Work out the finished part from the listing and answer in its coordinate system (mm). A direction names the side the tool comes from. Round coordinates to 2 decimals unless told otherwise and drop trailing zeros. Write each loop counter-clockwise with the first axis right and the second up, starting at its lowest first coordinate (ties: lowest second). Pieces come first, ordered by that corner, then holes. Notation, with made-up numbers: M 76,48.5 L 108,48.5 A19 ccw 108,54.5 Z; hole C -38.75,68.5 d9. An arc over 180 degrees is marked long. Answer in a Markdown table with one row per item.
```python
from build123d import *

# Parameters (mm, degrees)
BOSS_EXTRUDE1_DEPTH = 30
FILLET1_R           = 2
SHELL2_T            = 6
SKETCH3_R           = 9
CUT_EXTRUDE1_DEPTH  = 10
SKETCH4_R           = 9
CUT_EXTRUDE2_DEPTH  = 10
SKETCH5_R           = 9
CUT_EXTRUDE3_DEPTH  = 10
SKETCH7_R           = 4.5
CUT_EXTRUDE4_DEPTH  = 10
SKETCH8_R           = 4.5
CUT_EXTRUDE5_DEPTH  = 10
SKETCH9_R           = 4.5
CUT_EXTRUDE6_DEPTH  = 10
CHAMFER2_SIZE       = 2.5


with BuildPart() as part:
    # Sketch1 → Boss-Extrude1 (new body)
    with BuildSketch(Plane.XY):
        with BuildLine():
            Line((2, 0), (28, 0))
            ThreePointArc((28, 0), (29.414213562, 0.585786438), (30, 2))
            Line((30, 2), (30, 28))
            ThreePointArc((30, 28), (29.414213562, 29.414213562), (28, 30))
            Line((28, 30), (2, 30))
            ThreePointArc((2, 30), (0.585786438, 29.414213562), (0, 28))
            Line((0, 28), (0, 2))
            ThreePointArc((0, 2), (0.585786438, 0.585786438), (2, 0))
        make_face()
    extrude(amount=BOSS_EXTRUDE1_DEPTH)

    # Fillet1
    fillet1_edges = [part.edges().sort_by_distance(p)[0] for p in [
        (29.414213562, 0.585786438, 30),
        (15, 0, 0),
        (0.585786438, 0.585786438, 0),
        (30, 15, 30),
        (29.414213562, 29.414213562, 30),
        (15, 30, 30),
        (0.585786438, 29.414213562, 30),
        (0, 15, 30),
        (0.585786438, 0.585786438, 30),
        (15, 0, 30),
        (0, 15, 0),
        (0.585786438, 29.414213562, 0),
        (15, 30, 0),
        (29.414213562, 29.414213562, 0),
        (30, 15, 0),
        (29.414213562, 0.585786438, 0),
    ]]
    fillet(fillet1_edges, radius=FILLET1_R)

    # Shell2 (no face opened: a closed hollow body)
    add(offset(amount=-SHELL2_T, mode=Mode.PRIVATE), mode=Mode.SUBTRACT)

    # Sketch3 → Cut-Extrude1 (cut)
    with BuildSketch(Plane.XY.offset(30)):
        with Locations((15, 15)):
            Circle(SKETCH3_R)
    extrude(amount=-CUT_EXTRUDE1_DEPTH, mode=Mode.SUBTRACT)

    # Sketch4 → Cut-Extrude2 (cut)
    with BuildSketch(Plane(origin=(30, 0, 0), x_dir=(0, 0, -1), z_dir=(1, 0, 0))):
        with Locations((-15, 15)):
            Circle(SKETCH4_R)
    extrude(amount=-CUT_EXTRUDE2_DEPTH, mode=Mode.SUBTRACT)

    # Sketch5 → Cut-Extrude3 (cut)
    with BuildSketch(Plane(origin=(0, 30, 0), x_dir=(1, 0, 0), z_dir=(0, 1, 0))):
        with Locations(Location((15, -15, 0), (0, 0, 270))):
            Circle(SKETCH5_R)
    extrude(amount=-CUT_EXTRUDE3_DEPTH, mode=Mode.SUBTRACT)

    # Sketch7 → Cut-Extrude4 (cut)
    with BuildSketch(Plane.ZY):
        with Locations((15, 15)):
            Circle(SKETCH7_R)
    extrude(amount=-CUT_EXTRUDE4_DEPTH, mode=Mode.SUBTRACT)

    # Sketch8 → Cut-Extrude5 (cut)
    with BuildSketch(Plane(origin=(0, 0, 0), x_dir=(-1, 0, 0), z_dir=(0, 0, -1))):
        with Locations((-15, 15)):
            Circle(SKETCH8_R)
    extrude(amount=-CUT_EXTRUDE5_DEPTH, mode=Mode.SUBTRACT)

    # Sketch9 → Cut-Extrude6 (cut)
    with BuildSketch(Plane.XZ):
        with Locations(Location((15, 15, 0), (0, 0, 270))):
            Circle(SKETCH9_R)
    extrude(amount=-CUT_EXTRUDE6_DEPTH, mode=Mode.SUBTRACT)

    # Chamfer2
    # the kernel refuses this chamfer: 2.5 mm, written as the material it takes off along each edge
    with BuildSketch(Plane(origin=(6, 15, 15), x_dir=(0, 0, 1), z_dir=(0, -1, 0))) as chamfer2_piece_1:
        Polygon((4.5, CHAMFER2_SIZE), (4.5 + CHAMFER2_SIZE, 0), (4.5, 0), align=None)
    revolve(axis=Axis((6, 15, 15), (-1, 0, 0)), mode=Mode.SUBTRACT)
    with BuildSketch(Plane(origin=(15, 15, 6), x_dir=(-1, 0, 0), z_dir=(0, -1, 0))) as chamfer2_piece_2:
        Polygon((4.5, CHAMFER2_SIZE), (4.5 + CHAMFER2_SIZE, 0), (4.5, 0), align=None)
    revolve(axis=Axis((15, 15, 6), (0, 0, -1)), mode=Mode.SUBTRACT)
    with BuildSketch(Plane(origin=(15, 6, 15), x_dir=(0, 0, -1), z_dir=(-1, 0, 0))) as chamfer2_piece_3:
        Polygon((4.5, CHAMFER2_SIZE), (4.5 + CHAMFER2_SIZE, 0), (4.5, 0), align=None)
    revolve(axis=Axis((15, 6, 15), (0, -1, 0)), mode=Mode.SUBTRACT)


solid = part.part
```
1. Consider line 1 along Z through (x, y) = (22.75, 7.75); line 2 along Z through (x, y) = (16.5, 24.25). Determine where each line is inside the solid, lowest interval first. Write a range as from..to.
Calculated:
| item | result |
|---|---|
| line 1 | z = 0..6, 24..30 |
| line 2 | z = 0..6.13, 23.87..30 |
2. The part is cut by section C-C (y = 25). Determine the outline of the cut face in (x, z), plus the area to 3 significant figures.
Calculated:
| item | result |
|---|---|
| outline | M 0,2 A2 ccw 2,0 L 28,0 A2 ccw 30,2 L 30,28 A2 ccw 28,30 L 2,30 A2 ccw 0,28 Z; hole C 15,15 d18 |
| area | 642 mm² |
3. The part is cut by section D-D (y = 11.75). Count the separate pieces of the cut face and the enclosed holes in it, plus the area to 3 significant figures.
Calculated:
| item | result |
|---|---|
| separate pieces | 4 |
| enclosed holes | 0 |
| area | 280 mm² |
4. The part is cut by section B-B (x = 6.5). Determine the outline of the cut face in (y, z), plus the area to 3 significant figures.
Calculated:
| item | result |
|---|---|
| outline | M 0,2 A2 ccw 2,0 L 28,0 A2 ccw 30,2 L 30,12.04 L 24,12.04 L 24,6 L 6,6 L 6,24 L 12.04,24 L 12.04,30 L 2,30 A2 ccw 0,28 Z; M 17.96,24 L 24,24 L 24,17.96 L 30,17.96 L 30,28 A2 ccw 28,30 L 17.96,30 Z |
| area | 502 mm² |
5. The part is cut by section A-A (y = 3). Determine the outline of the cut face in (x, z).
Calculated:
| item | result |
|---|---|
| outline | M 0,2 A2 ccw 2,0 L 28,0 A2 ccw 30,2 L 30,28 A2 ccw 28,30 L 2,30 A2 ccw 0,28 Z; hole C 15,15 d9 |
6. A tool of negligible diameter and unlimited length cuts with its end or side. For faces 1 (the flat face through (22, 24, 22)), 2 (the cylindrical face through (17.703, 27.042, 23.584)), 3 (the cylindrical face through (23.584, 17.703, 27.042)), from which of +Z, -Z, +X, -X, +Y, -Y can it reach the whole face along a straight path? Write none if from no direction.
Calculated:
| item | result |
|---|---|
| face 1 | none |
| face 2 | +Y |
| face 3 | +Z |
7. Determine the mould class of faces 4 (the flat face through (22, 8, 24)), 5 (the conical face through (19, 4, 12)), 6 (the cylindrical face through (0.57, 14.82, 29.4)) for opening direction Y: released by +Y, released by -Y, zero draft, split by the parting line, or undercut.
Calculated:
| item | result |
|---|---|
| face 4 | undercut |
| face 5 | released by +Y |
| face 6 | zero draft |
8. Given pin 1 (9 mm diameter, centred on x = 15.5, y = 15.5, fed in from +Z); pin 2 (5.5 mm diameter, centred on y = 17, z = 13.5, fed in from +X); pin 3 (11 mm diameter, centred on x = 15, z = 15, fed in from +Y), each flat-ended and moving along its own axis, determine where each tip first touches the part or whether it passes through.
Calculated:
| item | result |
|---|---|
| pin 1 | stops at z = 4.21 |
| pin 2 | stops at x = 4.25 |
| pin 3 | stops at y = 4.5 |
